Can you work these out from the drawing? Everything is in mm from the part's minimum corner. A direction names the side the tool comes from. Round coordinates to 2 decimals unless told otherwise and drop trailing zeros. Loops run counter-clockwise (first coordinate to the right, second up) from the corner with the lowest first, then second, coordinate; pieces in that order, holes last. Notation, with made-up numbers: (44.25, -16) -> (50.25, -16) arc R21 cw to (50.25, -2) -> close; hole circle Ø11 at (20, -32). An arc over 180 degrees is marked (long way). Use CSV: the item, a comma, the result in double quotes. Start each with the question number.
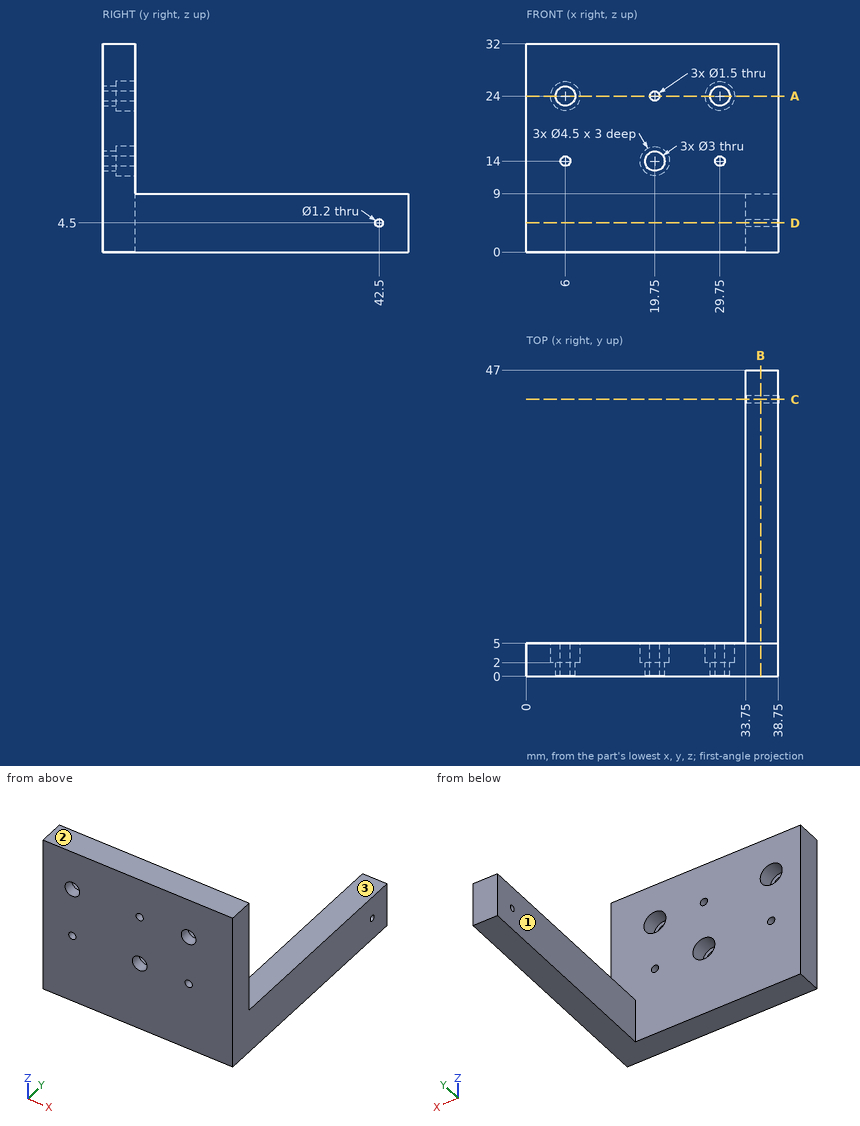
1. For the marked faces 1, 2 and 3, which set-ups out of +Z, -Z, +X, -X, +Y, -Y let a thin tool reach every point of the face, with its end or its side?
2. Suppose I cut it at D-D (z = 4.5). List the corners of the cut face in (x, y) for me.
3. If I drill on L1, parallel to X at y = 2.95, z = 14; L2, parallel to X at y = 3, z = 24; L3, parallel to Y at x = 26.5, z = 16, over which ranges is the centre line in solid material (lowest first)?
4. Suppose I cut it at C-C (y = 42.5). List the corners of the cut face in (x, z) for me, then the cut area to 3 significant figures.
5. Suppose I cut it at B-B (x = 36). List the corners of the cut face in (y, z) for me.
6. Suppose I cut it at A-A (z = 24). List the corners of the cut face in (x, y) for me.
7. Will these pins go through, and if not, where does the flat tip stop? pin 1 (2 mm diameter, centred on x = 30, z = 23, fed in from +Y); pin 2 (1 mm diameter, centred on y = 42.5, z = 4.5, fed in from -X); pin 3 (2.5 mm diameter, centred on x = 35.5, y = 17, fed in from +Z); pin 4 (7 mm diameter, centred on x = 6, z = 24, fed in from +Y).
Geometry check:
1,face 1,"+Z, -Z, -X, +Y"
1,face 2,"+Z, +X, -X, +Y, -Y"
1,face 3,"+Z, +X, -X, +Y"
2,outline,"(0, 0) -> (38.75, 0) -> (38.75, 41.9) -> (33.75, 41.9) -> (33.75, 5) -> (0, 5) -> close; (33.75, 43.1) -> (38.75, 43.1) -> (38.75, 47) -> (33.75, 47) -> close"
3,L1,"x = 0 to 5.25, 6.75 to 17.5, 22 to 29, 30.5 to 38.75"
3,L2,"x = 0 to 3.75, 8.25 to 19, 20.5 to 27.5, 32 to 38.75"
3,L3,"y = 0 to 5"
4,outline,"(33.75, 0) -> (38.75, 0) -> (38.75, 3.9) -> (33.75, 3.9) -> close; (33.75, 5.1) -> (38.75, 5.1) -> (38.75, 9) -> (33.75, 9) -> close"
4,area,"39.0 mm²"
5,outline,"(0, 0) -> (47, 0) -> (47, 9) -> (5, 9) -> (5, 32) -> (0, 32) -> close; hole circle Ø1.2 at (42.5, 4.5)"
6,outline,"(0, 0) -> (4.5, 0) -> (4.5, 2) -> (3.75, 2) -> (3.75, 5) -> (0, 5) -> close; (7.5, 0) -> (19, 0) -> (19, 5) -> (8.25, 5) -> (8.25, 2) -> (7.5, 2) -> close; (20.5, 0) -> (28.25, 0) -> (28.25, 2) -> (27.5, 2) -> (27.5, 5) -> (20.5, 5) -> close; (31.25, 0) -> (38.75, 0) -> (38.75, 5) -> (32, 5) -> (32, 2) -> (31.25, 2) -> close"
7,pin 1,"stops at y = 2"
7,pin 2,"passes through"
7,pin 3,"stops at z = 9"
7,pin 4,"stops at y = 5"
